```python
from build123d import *

# Parameters (mm, degrees)
SKETCH1_R           = 1.7
BOSS_EXTRUDE1_DEPTH = 5
CUT_EXTRUDE1_START  = -5
CUT_EXTRUDE1_DEPTH  = 4
BOSS_EXTRUDE3_DEPTH = 4.5
BOSS_EXTRUDE4_DEPTH = 0.75


with BuildPart() as part:
    # Sketch1 → Boss-Extrude1 (new body)
    with BuildSketch(Plane(origin=(0, 0, 0), x_dir=(1, 0, 0), z_dir=(0, 1, 0))):
        with BuildLine():
            Line((-4.494644994, 13.719468408), (-4.772250922, 8.034184997))
            ThreePointArc((-4.772250922, 8.034184997), (-6.10009687, 3.52189257), (-9.343933767, 0.115798034))
            Line((-9.343933767, 0.115798034), (-14.128730664, -2.967257459))
            ThreePointArc((-14.128730664, -2.967257459), (-15.588457268, -9), (-9.634085671, -10.752210949))
            Line((-9.634085671, -10.752210949), (-4.571682845, -8.149983031))
            ThreePointArc((-4.571682845, -8.149983031), (0, -7.04378514), (4.571682845, -8.149983031))
            Line((4.571682845, -8.149983031), (9.634085671, -10.752210949))
            ThreePointArc((9.634085671, -10.752210949), (15.588457268, -9), (14.128730664, -2.967257459))
            Line((14.128730664, -2.967257459), (9.343933767, 0.115798034))
            ThreePointArc((9.343933767, 0.115798034), (6.10009687, 3.52189257), (4.772250922, 8.034184997))
            Line((4.772250922, 8.034184997), (4.494644994, 13.719468408))
            ThreePointArc((4.494644994, 13.719468408), (0, 18), (-4.494644994, 13.719468408))
        make_face()
        with Locations((0, 13.5)):
            Circle(SKETCH1_R, mode=Mode.SUBTRACT)
        with Locations((11.691342951, -6.75)):
            Circle(SKETCH1_R, mode=Mode.SUBTRACT)
        with Locations((-11.691342951, -6.75)):
            Circle(SKETCH1_R, mode=Mode.SUBTRACT)
    extrude(amount=BOSS_EXTRUDE1_DEPTH)

    # Sketch2 → Cut-Extrude1 (cut)
    with BuildSketch(Plane(origin=(0, 5, 0), x_dir=(1, 0, 0), z_dir=(0, 1, 0)).offset(CUT_EXTRUDE1_START)):
        Polygon((14.441342951, -8.33771324), (14.441342951, -5.16228676), (11.691342951, -3.574573519), (8.941342951, -5.16228676), (8.941342951, -8.33771324), (11.691342951, -9.925426481), align=None)
        Polygon((0, 16.675426481), (-2.75, 15.08771324), (-2.75, 11.91228676), (0, 10.324573519), (2.75, 11.91228676), (2.75, 15.08771324), align=None)
        Polygon((-14.441342951, -8.33771324), (-11.691342951, -9.925426481), (-8.941342951, -8.33771324), (-8.941342951, -5.16228676), (-11.691342951, -3.574573519), (-14.441342951, -5.16228676), align=None)
    extrude(amount=CUT_EXTRUDE1_DEPTH, mode=Mode.SUBTRACT)

    # Sketch7 → Boss-Extrude3 (add)
    with BuildSketch(Plane.XZ):
        with BuildLine():
            ThreePointArc((-4.872953171, -7.025441438), (0, -8.55), (4.872953171, -7.025441438))
            ThreePointArc((4.872953171, -7.025441438), (6.10009687, -3.52189257), (8.520687343, -0.707380519))
            ThreePointArc((8.520687343, -0.707380519), (7.404517202, 4.275), (3.647734172, 7.732821956))
            ThreePointArc((3.647734172, 7.732821956), (0, 7.04378514), (-3.647734172, 7.732821956))
            ThreePointArc((-3.647734172, 7.732821956), (-7.404517202, 4.275), (-8.520687343, -0.707380519))
            ThreePointArc((-8.520687343, -0.707380519), (-6.10009687, -3.52189257), (-4.872953171, -7.025441438))
        make_face()
    extrude(amount=BOSS_EXTRUDE3_DEPTH)

    # Sketch8 → Boss-Extrude4 (add)
    with BuildSketch(Plane.XZ):
        with BuildLine():
            Line((-9.343933767, -0.115798034), (-9.499987767, -0.015245565))
            ThreePointArc((-9.499987767, -0.015245565), (-8.227241336, 4.75), (-4.736790837, 8.234853524))
            Line((-4.736790837, 8.234853524), (-4.571682845, 8.149983031))
            ThreePointArc((-4.571682845, 8.149983031), (-4.114998161, 7.929686713), (-3.647734172, 7.732821956))
            ThreePointArc((-3.647734172, 7.732821956), (-7.404517202, 4.275), (-8.520687343, -0.707380519))
            ThreePointArc((-8.520687343, -0.707380519), (-8.924809218, -0.401150413), (-9.343933767, -0.115798034))
        make_face()
        with BuildLine():
            Line((4.571682845, 8.149983031), (4.736790837, 8.234853524))
            ThreePointArc((4.736790837, 8.234853524), (8.227241336, 4.75), (9.499987767, -0.015245565))
            Line((9.499987767, -0.015245565), (9.343933767, -0.115798034))
            ThreePointArc((9.343933767, -0.115798034), (8.924809218, -0.401150413), (8.520687343, -0.707380519))
            ThreePointArc((8.520687343, -0.707380519), (7.404517202, 4.275), (3.647734172, 7.732821956))
            ThreePointArc((3.647734172, 7.732821956), (4.114998161, 7.929686713), (4.571682845, 8.149983031))
        make_face()
        with BuildLine():
            Line((4.772250922, -8.034184997), (4.76319693, -8.219607959))
            ThreePointArc((4.76319693, -8.219607959), (0, -9.5), (-4.76319693, -8.219607959))
            Line((-4.76319693, -8.219607959), (-4.772250922, -8.034184997))
            ThreePointArc((-4.772250922, -8.034184997), (-4.809811057, -7.528536301), (-4.872953171, -7.025441437))
            ThreePointArc((-4.872953171, -7.025441437), (0, -8.55), (4.872953171, -7.025441438))
            ThreePointArc((4.872953171, -7.025441438), (4.809811057, -7.528536301), (4.772250922, -8.034184997))
        make_face()
    extrude(amount=BOSS_EXTRUDE4_DEPTH)


solid = part.part
```
Input: part model. Units: mm. Frame: model coordinates. A direction names the side the tool comes from. Give positions to 0.01 mm unless a question says otherwise; leave off trailing zeros. Order: outer loops, then holes, each group sorted by start corner. A loop starts at its lowest first (then second) coordinate and runs counter-clockwise, first axis right, second up.
1. Section C-C on x = 11. Return the cut outline in (y, z).
Derived:
outline: (0, 0.95) - (5, 0.95) - (5, 5.2) - (4, 5.2) - (4, 3.97) - (0, 3.97) - close; (0, 9.53) - (4, 9.53) - (4, 8.3) - (5, 8.3) - (5, 11.2) - (0, 11.2) - close
2. Reachability of faces 1 (the flat face through (-8.941, 2, 7)), 2 (the flat face through (0, -4.5, 0)), 3 (the cylindrical face through (-0.07, -2.6, -8.55)) from +Z, -Z, +X, -X, +Y, -Y: full face, straight path, thin tool, end or side. Return the list, or none.
Derived:
face 1: -Y
face 2: +Z, -Z, +X, -X, -Y
face 3: -Z, -Y
3. Section B-B on z = 4.25. Return the cut outline in (x, y), and give its area (3 significant figures).
Derived:
outline: (-15.43, 0) - (-12.86, 0) - (-12.86, 4) - (-10.52, 4) - (-10.52, 0) - (-8.5, 0) - (-8.5, -0.75) - (-7.42, -0.75) - (-7.42, -4.5) - (7.42, -4.5) - (7.42, -0.75) - (8.5, -0.75) - (8.5, 0) - (10.52, 0) - (10.52, 4) - (12.86, 4) - (12.86, 0) - (15.43, 0) - (15.43, 5) - (-15.43, 5) - close
area: 204 mm2
4. Mould query, pull axis Z, two halves, no side actions, for faces 4 (the flat face through (8, -0.75, 4)), 5 (the flat face through (10.3, 1.97, 9.12)), 6 (the cylindrical face through (0.1, -0.4, -9.5)). Classes: released by +Z, released by -Z, zero draft, split by the parting line, or undercut.
Derived:
face 4: zero draft
face 5: undercut
face 6: released by -Z
5. Material intervals for L1, parallel to X at y = 4.45, z = 6.75; L2, parallel to Y at x = 10, z = 7.5; L3, parallel to Z at x = 11, y = 1, sorted ascending.
Derived:
L1: x = -16.19 to -13.39, -9.99 to 9.99, 13.39 to 16.19
L2: y = 4 to 5
L3: z = 0.95 to 3.97, 9.53 to 11.2
6. Pin query (flat end, axial travel): pin 1 (3 mm diameter, centred on x = -0.5, z = -12.5, fed in from -Y); pin 2 (2.5 mm diameter, centred on y = 2.5, z = -13.5, fed in from +X); pin 3 (4 mm diameter, centred on y = 4, z = -5.5, fed in from -X). Return the tip coordinate at first contact, or that it passes through.
Derived:
pin 1: stops at y = 4
pin 2: stops at x = 4.57
pin 3: stops at x = -6.11
7. Section A-A on x = 1. Return the cut outline in (y, z), and give its area (3 significant figures).
Derived:
outline: (-4.5, -8.49) - (-0.75, -8.49) - (-0.75, -9.45) - (0, -9.45) - (0, -10.9) - (4, -10.9) - (4, -12.13) - (5, -12.13) - (5, 7.09) - (-4.5, 7.09) - close; (0, -17.89) - (5, -17.89) - (5, -14.87) - (4, -14.87) - (4, -16.1) - (0, -16.1) - close
area: 172 mm2
